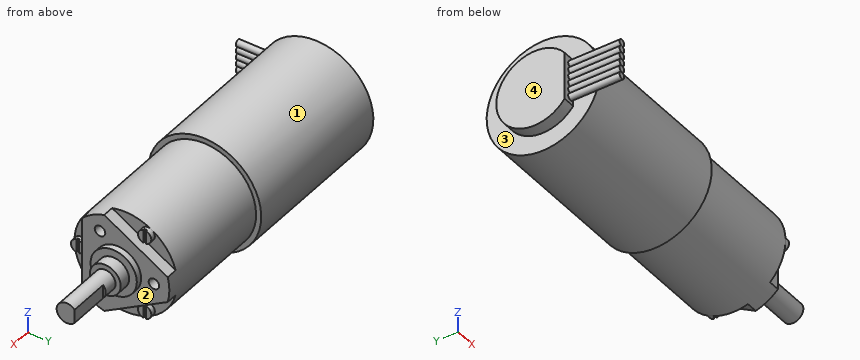
```python
from build123d import *

# Parameters (mm, degrees)
TROU_TARAUD_M2_51_D          = 2.05
TROU_TARAUD_M2_51_DEPTH      = 4.35
TROU_TARAUD_M2_51_TIP        = 0.615882135
ENL_V_START                  = -2.2
ENL_V_MAT_EXTRU_1_DEPTH      = 2.2
ESQUISSE5_R                  = 1.3
BOSS_EXTRU_1_DEPTH           = 1
ESQUISSE6_W                  = 2.6
ESQUISSE6_H                  = 0.5
ENL_V_MAT_EXTRU_2_DEPTH      = 0.3
ENL_V_MAT_EXTRU_3_DEPTH      = 72.707740168
ENL_V_MAT_EXTRU_3_DEPTH_BACK = 72.707740168
ESQUISSE7_W                  = 8
ESQUISSE7_H                  = 0.5
BOSS_EXTRU_2_DEPTH           = 2.4
ESQUISSE9_R                  = 0.65
BOSS_EXTRU_3_DEPTH           = 10


with BuildPart() as part:
    # Esquisse1 → Révolution1 (revolve)
    with BuildSketch(Plane.XY, mode=Mode.PRIVATE) as r_volution1_sk:
        Polygon((70, 0), (70, 2), (59.25, 2), (59.25, 3), (56.9, 3), (56.9, 4.5), (55.7, 4.5), (55.7, 10), (31.4, 10), (31.4, 11), (0, 11), (0, 0), align=None)
    revolve(r_volution1_sk.sketch.rotate(Axis((0, 0, 0), (1, 0, 0)), 90), axis=Axis((0, 0, 0), (1, 0, 0)))

    # Trou taraudé M2.51
    with Locations(Plane(origin=(55.7, 0, 0), x_dir=(0, 0, -1), z_dir=(1, 0, 0))):
        with Locations((0, 7), (-6.062177826, -3.5), (6.062177826, -3.5)):
            Hole(TROU_TARAUD_M2_51_D / 2, depth=TROU_TARAUD_M2_51_DEPTH)
            with Locations((0, 0, -(TROU_TARAUD_M2_51_DEPTH + TROU_TARAUD_M2_51_TIP / 2))):  # 118° drill point
                Cone(0, TROU_TARAUD_M2_51_D / 2, TROU_TARAUD_M2_51_TIP, mode=Mode.SUBTRACT)

    # Esquisse4 → Enlèv. mat.-Extru.1 (cut)
    with BuildSketch(Plane(origin=(55.7, 0, 0), x_dir=(0, 0, -1), z_dir=(1, 0, 0)).offset(ENL_V_START)):
        with BuildLine():
            Line((-9.632892041, -2.684658438), (-2.491463612, 9.684658438))
            ThreePointArc((-2.491463612, 9.684658438), (-8.660254038, 5), (-9.632892041, -2.684658438))
        make_face()
        with BuildLine():
            Line((0, -7), (-7.141428429, -7))
            ThreePointArc((-7.141428429, -7), (-3.872983346, -9.219544457), (0, -10))
            Line((0, -10), (0, -7))
        make_face()
        with BuildLine():
            ThreePointArc((0, -10), (3.872983346, -9.219544457), (7.141428429, -7))
            Line((7.141428429, -7), (0, -7))
            Line((0, -7), (0, -10))
        make_face()
        with BuildLine():
            ThreePointArc((10, 0), (7.902994247, 6.127208332), (2.491463612, 9.684658438))
            Line((2.491463612, 9.684658438), (9.632892041, -2.684658438))
            ThreePointArc((9.632892041, -2.684658438), (9.907797949, -1.354820946), (10, 0))
        make_face()
    extrude(amount=ENL_V_MAT_EXTRU_1_DEPTH, mode=Mode.SUBTRACT)

    # Esquisse5 → Boss.-Extru.1 (add)
    with BuildSketch(Plane(origin=(53.5, 0, 0), x_dir=(0, 0, -1), z_dir=(1, 0, 0))):
        with Locations(Location((-7.534421013, 4.35, 0), (0, 0, 149.999238117))):
            Circle(ESQUISSE5_R)
        with Locations(Location((7.534421013, 4.35, 0), (0, 0, 29.999238117))):
            Circle(ESQUISSE5_R)
        with Locations(Location((0, -8.7, 0), (0, 0, 269.999238081))):
            Circle(ESQUISSE5_R)
    extrude(amount=BOSS_EXTRU_1_DEPTH)

    # Esquisse6 → Enlèv. mat.-Extru.2 (cut)
    with BuildSketch(Plane(origin=(54.5, 0, 0), x_dir=(0, 0, -1), z_dir=(1, 0, 0))):
        with Locations((-7.534421013, 4.35)):
            Rectangle(ESQUISSE6_W, ESQUISSE6_H)
        with Locations((7.534421013, 4.35)):
            Rectangle(ESQUISSE6_W, ESQUISSE6_H)
        with Locations((0, -8.7)):
            Rectangle(ESQUISSE6_W, ESQUISSE6_H)
    extrude(amount=-ENL_V_MAT_EXTRU_2_DEPTH, mode=Mode.SUBTRACT)

    # Esquisse7 → Enlèv. mat.-Extru.3 (cut, two sides: drawn at the far end of the back side and taken through both)
    with BuildSketch(Plane.XY.offset(-ENL_V_MAT_EXTRU_3_DEPTH_BACK)):
        with Locations((66, 1.75)):
            Rectangle(ESQUISSE7_W, ESQUISSE7_H)
    extrude(amount=ENL_V_MAT_EXTRU_3_DEPTH + ENL_V_MAT_EXTRU_3_DEPTH_BACK, mode=Mode.SUBTRACT)

    # Esquisse8 → Boss.-Extru.2 (add)
    with BuildSketch(Plane.ZY):
        with BuildLine():
            Line((-4.613025038, -5.85), (4.613025038, -5.85))
            ThreePointArc((4.613025038, -5.85), (0, 7.45), (-4.613025038, -5.85))
        make_face()
    extrude(amount=BOSS_EXTRU_2_DEPTH)

    # Esquisse9 → Boss.-Extru.3 (add)
    with BuildSketch(Plane.XZ.offset(5.85)):
        with Locations(Location((-0.75, 3.275, 0), (0, 0, 90))):
            Circle(ESQUISSE9_R)
        with Locations(Location((-0.75, 1.965, 0), (0, 0, 90))):
            Circle(ESQUISSE9_R)
        with Locations(Location((-0.75, 0.655, 0), (0, 0, 90))):
            Circle(ESQUISSE9_R)
        with Locations(Location((-0.75, -0.655, 0), (0, 0, 90))):
            Circle(ESQUISSE9_R)
        with Locations(Location((-0.75, -1.965, 0), (0, 0, 90))):
            Circle(ESQUISSE9_R)
        with Locations(Location((-0.75, -3.275, 0), (0, 0, 90))):
            Circle(ESQUISSE9_R)
    extrude(amount=BOSS_EXTRU_3_DEPTH)


solid = part.part
```
Geometry: final body of the model. Coordinates: model frame, mm. Face numbers are marked on the shaded views. Coordinates: 2 decimals unless noted, no trailing zeros. Order: outer loops, then holes, each group sorted by start corner. A loop starts at its lowest first (then second) coordinate and runs counter-clockwise, first axis right, second up. Notation, with made-up numbers: (39.25, -19) - (68.25, -19) arc R8 ccw to (68.25, -5) - close; hole circle Ø1 at (51, 78.5). An arc over 180 degrees is marked (long way). Return JSON: item names as keys, results as strings. Group by question number.
1. Pull-direction query (X, two-part tool) for the marked faces 1, 2, 3 and 4; classes: pulls with the +X half, pulls with the -X half, needs draft (parallel to the pull), parting line crosses it, or undercut.
2. Cut plane B-B (y = 0). Output: boundary loops of the cut face in (x, z), plus the area to 3 significant figures.
3. Pin query (flat end, axial travel): pin 1 (4 mm diameter, centred on y = -11, z = -1.5, fed in from +X); pin 2 (10 mm diameter, centred on x = 56.5, y = 4, fed in from -Z); pin 3 (10 mm diameter, centred on x = 37, y = 2.5, fed in from +Z). Return the tip coordinate at first contact, or that it passes through.
4. Cut plane C-C (x = 38.5). Output: boundary loops of the cut face in (y, z).
5. Cut plane D-D (x = 16). Output: boundary loops of the cut face in (y, z).
6. Cut plane A-A (x = -0.75). Output: boundary loops of the cut face in (y, z) (3 decimals), plus the area to 3 significant figures.
7. Material intervals for line 1 along Y through (x, z) = (52.6, 0) (3 decimals); line 2 along Z through (x, y) = (53.25, -3.5); line 3 along Z through (x, y) = (52.5, 7) (3 decimals), sorted ascending. Write a range as [from, to].
Resolved:
{
 "1": {"face 1": "needs draft", "face 2": "pulls with the +X half", "face 3": "undercut", "face 4": "pulls with the -X half"},
 "2": {"outline": "(-2.4, -7.45) - (0, -7.45) - (0, -11) - (31.4, -11) - (31.4, -10) - (53.5, -10) - (53.5, -8.08) - (55.7, -8.08) - (55.7, -4.5) - (56.9, -4.5) - (56.9, -3) - (59.25, -3) - (59.25, -2) - (70, -2) - (70, 2) - (59.25, 2) - (59.25, 3) - (56.9, 3) - (56.9, 4.5) - (55.7, 4.5) - (55.7, 8.08) - (53.5, 8.08) - (53.5, 10) - (31.4, 10) - (31.4, 11) - (0, 11) - (0, 7.45) - (-2.4, 7.45) - close", "area": "1,270 mm²"},
 "3": {"pin 1": "stops at x = 54.5", "pin 2": "stops at z = -10", "pin 3": "stops at z = 10"},
 "4": {"outline": "circle Ø20 at (0, 0)"},
 "5": {"outline": "circle Ø22 at (0, 0)"},
 "6": {"outline": "(-15.85, -3.925) - (-5.85, -3.925) - (-5.85, -4.613) arc R7.45 ccw (long way) to (-5.85, 4.613) - (-5.85, 3.925) - (-15.85, 3.925) - (-15.85, 2.625) - (-5.85, 2.625) - (-5.85, 2.615) - (-15.85, 2.615) - (-15.85, 1.315) - (-5.85, 1.315) - (-5.85, 1.305) - (-15.85, 1.305) - (-15.85, 0.005) - (-5.85, 0.005) - (-5.85, -0.005) - (-15.85, -0.005) - (-15.85, -1.305) - (-5.85, -1.305) - (-5.85, -1.315) - (-15.85, -1.315) - (-15.85, -2.615) - (-5.85, -2.615) - (-5.85, -2.625) - (-15.85, -2.625) - close", "area": "242 mm²"},
 "7": {"line 1": "y = [-10, 5.975], [8.025, 10]", "line 2": "z = [-9.37, -7.09], [-5.04, 5.04], [7.09, 9.37]", "line 3": "z = [-7.141, -1.025], [1.025, 7.141]"}
}
